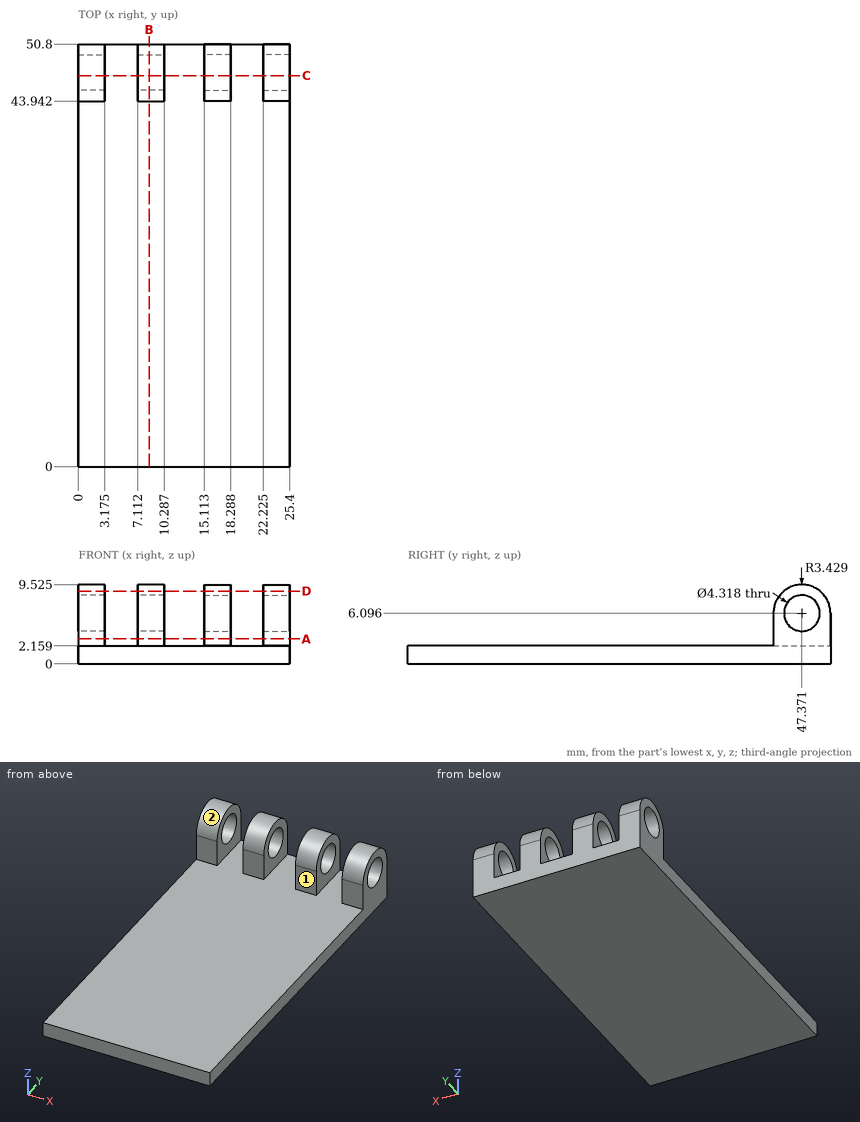
Source: three-view drawing plus pictorial views. Frame: mm from the lowest corner of the part. A direction names the side the tool comes from. Coordinates: 2 decimals unless noted, no trailing zeros. Order: outer loops, then holes, each group sorted by start corner. A loop starts at its lowest first (then second) coordinate and runs counter-clockwise, first axis right, second up.
1) Section A-A (z = 3). Return loops of the section in (x, y) (3 decimals).
Result sheet:
outline: (0, 43.942) - (3.175, 43.942) - (3.175, 50.8) - (0, 50.8) - close; (7.112, 43.942) - (10.287, 43.942) - (10.287, 50.8) - (7.112, 50.8) - close; (15.113, 43.942) - (18.288, 43.942) - (18.288, 50.8) - (15.113, 50.8) - close; (22.225, 43.942) - (25.4, 43.942) - (25.4, 50.8) - (22.225, 50.8) - close
2) Section B-B (x = 8.5). Return loops of the section in (y, z).
Result sheet:
outline: (0, 0) - (50.8, 0) - (50.8, 6.1) arc R3.43 ccw to (43.94, 6.1) - (43.94, 2.16) - (0, 2.16) - close; hole circle Ø4.32 at (47.37, 6.1)
3) Section D-D (z = 8.75). Return loops of the section in (x, y) (3 decimals).
Result sheet:
outline: (0, 45.2) - (3.175, 45.2) - (3.175, 49.542) - (0, 49.542) - close; (7.112, 45.2) - (10.287, 45.2) - (10.287, 49.542) - (7.112, 49.542) - close; (15.113, 45.2) - (18.288, 45.2) - (18.288, 49.542) - (15.113, 49.542) - close; (22.225, 45.2) - (25.4, 45.2) - (25.4, 49.542) - (22.225, 49.542) - close
4) Ray query, probe 1 along Z at (x, y) = (9, 27); probe 2 along Y at (x, z) = (9, 3); probe 3 along Y at (x, z) = (10, 7). Return the intervals inside material, ascending.
Result sheet:
probe 1: z = 0 to 2.16
probe 2: y = 43.94 to 50.8
probe 3: y = 44.06 to 45.41, 49.33 to 50.68
5) First-contact query: P1, Ø12.5, axis at x = 8, y = 29.5, coming from the +Z side; P2, Ø1, axis at x = 8.5, z = 5, coming from the -Y side. Flat tips, straight axial feed; report the tip coordinate or a pass-through.
Result sheet:
P1: stops at z = 2.16
P2: stops at y = 43.94
6) Set-up query: the marked faces 1 and 2. Return all of +Z, -Z, +X, -X, +Y, -Y with unobstructed straight access to the full face (end or side cutting, diameter ignored); none if empty.
Result sheet:
face 1: +Z, +X, -X, -Y
face 2: +Z, +X, -X
7) Section C-C (y = 47). Give the number of separate pieces and of enclosed holes in the cut face, then the cut area to 3 significant figures.
Result sheet:
separate pieces: 5
enclosed holes: 0
area: 94.1 mm2
